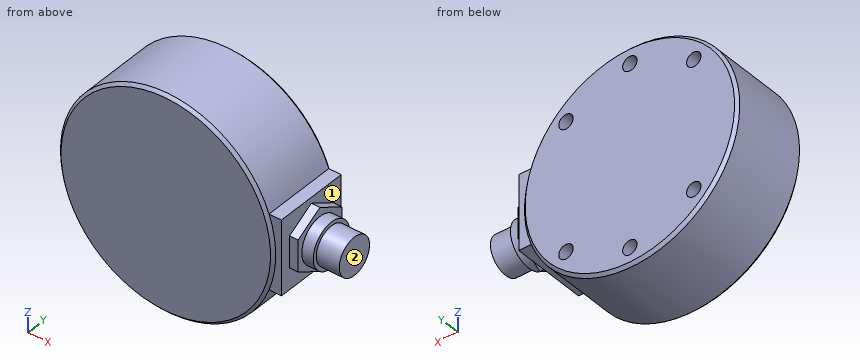
from build123d import *

# Parameters (mm, degrees)
SKETCH1_R           = 37.5
BOSS_EXTRUDE1_DEPTH = 28
CHAMFER1_SIZE       = 1
BOSS_EXTRUDE2_REACH = 92.107
SKETCH2_W           = 26
SKETCH2_H           = 26
BOSS_EXTRUDE3_DEPTH = 3
SKETCH4_R           = 7.9
BOSS_EXTRUDE4_DEPTH = 4
SKETCH5_R           = 6.58
BOSS_EXTRUDE5_DEPTH = 8
SKETCH6_R           = 2.5
CUT_EXTRUDE1_DEPTH  = 5


with BuildPart() as part:
    # Sketch1 → Boss-Extrude1 (new body)
    with BuildSketch(Plane(origin=(0, 0, 0), x_dir=(1, 0, 0), z_dir=(0, 1, 0))):
        with Locations(Location((0, 0, 0), (0, 0, 270))):
            Circle(SKETCH1_R)
    extrude(amount=BOSS_EXTRUDE1_DEPTH)

    # Chamfer1
    chamfer1_edges = [part.edges().sort_by_distance(p)[0] for p in [
        (0, 0, -37.5),
        (0, 28, -37.5),
    ]]
    chamfer(chamfer1_edges, length=CHAMFER1_SIZE)

    # Sketch2 → Boss-Extrude2 (add, up to next)
    with BuildSketch(Plane(origin=(39.5, 0, 0), x_dir=(0, 0, -1), z_dir=(1, 0, 0)), mode=Mode.PRIVATE) as boss_extrude2_sk1:
        with Locations((0, 14)):
            Rectangle(SKETCH2_W, SKETCH2_H)
    boss_extrude2_tool1 = extrude(boss_extrude2_sk1.sketch, amount=-BOSS_EXTRUDE2_REACH, mode=Mode.PRIVATE) - part.part
    add(boss_extrude2_tool1.solids().sort_by_distance((39.5, 14, 0))[0])

    # Sketch3 → Boss-Extrude3 (add)
    with BuildSketch(Plane(origin=(39.5, 0, 0), x_dir=(0, 0, -1), z_dir=(1, 0, 0))):
        Polygon((10.97, 14), (5.485, 23.50029868), (-5.485, 23.50029868), (-10.97, 14), (-5.485, 4.49970132), (5.485, 4.49970132), align=None)
    extrude(amount=BOSS_EXTRUDE3_DEPTH)

    # Sketch4 → Boss-Extrude4 (add)
    with BuildSketch(Plane(origin=(42.5, 0, 0), x_dir=(0, 0, -1), z_dir=(1, 0, 0))):
        with Locations((0, 14)):
            Circle(SKETCH4_R)
    extrude(amount=BOSS_EXTRUDE4_DEPTH)

    # Sketch5 → Boss-Extrude5 (add)
    with BuildSketch(Plane(origin=(46.5, 0, 0), x_dir=(0, 0, -1), z_dir=(1, 0, 0))):
        with Locations((0, 14)):
            Circle(SKETCH5_R)
    extrude(amount=BOSS_EXTRUDE5_DEPTH)

    # Sketch6 → Cut-Extrude1 (cut)
    with BuildSketch(Plane(origin=(0, 28, 0), x_dir=(1, 0, 0), z_dir=(0, 1, 0))):
        with Locations(Location((0, 31.5, 0), (0, 0, 270))):
            Circle(SKETCH6_R)
        with Locations(Location((0, -31.5, 0), (0, 0, 270))):
            Circle(SKETCH6_R)
        with Locations(Location((22.27, -22.277726545, 0), (0, 0, 270))):
            Circle(SKETCH6_R)
        with Locations(Location((-22.27, -22.277726545, 0), (0, 0, 270))):
            Circle(SKETCH6_R)
        with Locations(Location((-22.27, 22.277726545, 0), (0, 0, 270))):
            Circle(SKETCH6_R)
        with Locations(Location((22.27, 22.277726545, 0), (0, 0, 270))):
            Circle(SKETCH6_R)
    extrude(amount=-CUT_EXTRUDE1_DEPTH, mode=Mode.SUBTRACT)


solid = part.part
Work out the finished part from the listing and answer in its coordinate system (mm). Face numbers are marked on the shaded views. A direction names the side the tool comes from. Give positions to 0.01 mm unless a question says otherwise; leave off trailing zeros. Order: outer loops, then holes, each group sorted by start corner. A loop starts at its lowest first (then second) coordinate and runs counter-clockwise, first axis right, second up. Notation, with made-up numbers: (-21, 23) -> (-1, 23) arc R20 ccw to (-1, 37) -> close; hole circle Ø9 at (-12, 5). An arc over 180 degrees is marked (long way). Answer as a JSON object with one key per item and string values. Group by question number.
1. Section A-A on x = 0 is taken. Determine the outline of the cut face in (y, z).
2. Section B-B on y = 10 is taken. Determine the outline of the cut face in (x, z).
3. A tool of negligible diameter and unlimited length cuts with its end or side. For the marked faces 1 and 2, from which of +Z, -Z, +X, -X, +Y, -Y can it reach the whole face along a straight path? Write none if from no direction.
4. Flat-ended cylindrical pins translate along their axes: pin 1 Ø3 at (x, z) = (0, 31.5) entering from +Y; pin 2 Ø1.5 at (x, z) = (41.5, 0.5) entering from -Y; pin 3 Ø1.5 at (y, z) = (7.5, -21) entering from -X. Find the tip coordinate at first contact, or state that the pin passes through.
5. Consider line 1 along Z through (x, y) = (0.5, 18.5); line 2 along Z through (x, y) = (22.5, 24.25); line 3 along X through (y, z) = (26.1, -31.5). Determine where each line is inside the solid, lowest interval first. Write a range as [from, to].
6. Section C-C on y = 2.75 is taken. Determine the outline of the cut face in (x, z).
Result sheet:
{
 "1": {"outline": "(0, -36.5) -> (1, -37.5) -> (27, -37.5) -> (28, -36.5) -> (28, -34) -> (23, -34) -> (23, -29) -> (28, -29) -> (28, 29) -> (23, 29) -> (23, 34) -> (28, 34) -> (28, 36.5) -> (27, 37.5) -> (1, 37.5) -> (0, 36.5) -> close"},
 "2": {"outline": "(35.17, -13) -> (39.5, -13) -> (39.5, -8.66) -> (42.5, -8.66) -> (42.5, -6.81) -> (46.5, -6.81) -> (46.5, -5.22) -> (54.5, -5.22) -> (54.5, 5.22) -> (46.5, 5.22) -> (46.5, 6.81) -> (42.5, 6.81) -> (42.5, 8.66) -> (39.5, 8.66) -> (39.5, 13) -> (35.17, 13) arc R37.5 ccw (long way) to start"},
 "3": {"face 1": "+X", "face 2": "+Z, -Z, +X, +Y, -Y"},
 "4": {"pin 1": "stops at y = 23", "pin 2": "stops at y = 4.5", "pin 3": "stops at x = -31.56"},
 "5": {"line 1": "z = [-37.5, 37.5]", "line 2": "z = [-30, -24.77], [-19.79, 19.79], [24.77, 30]", "line 3": "x = [-20.35, -2.5], [2.5, 20.35]"},
 "6": {"outline": "(35.17, -13) -> (39.5, -13) -> (39.5, 13) -> (35.17, 13) arc R37.5 ccw (long way) to start"}
}
